from build123d import *

# Parameters (mm, degrees)
F0_W      = 25
F0_H      = 45
F1_DEPTH  = 25
F3_DEPTH  = 25
F5_DEPTH  = 25
F6_W      = 5
F6_H      = 12
F7_DEPTH  = 12
F9_DEPTH  = 25
F10_R     = 5
F11_W     = 5
F11_H     = 12
F12_DEPTH = 12
F14_DEPTH = 25
F15_R     = 5
F16_W     = 19
F16_H     = 6
F17_DEPTH = 19
F19_DEPTH = 12
F20_R     = 5
F21_R     = 5
F22_DEPTH = 2
F23_DEPTH = 19
F24_DEPTH = 7


with BuildPart() as f1:
    # F0 (on Front) → F1 (new body)
    with BuildSketch(Plane.XZ):
        with Locations((12.5, 22.5)):
            Rectangle(F0_W, F0_H)
    extrude(amount=F1_DEPTH)

    # F2 (on face) → F3 (cut)
    with BuildSketch(Plane.XZ.offset(25)):
        with BuildLine():
            ThreePointArc((16.5, 25), (9.6715728753, 27.8284271247), (12.5, 21))
            ThreePointArc((12.5, 21), (15.3284271247, 22.1715728753), (16.5, 25))
        make_face()
    extrude(amount=-F3_DEPTH, mode=Mode.SUBTRACT)

    # F4 (on face) → F5 (cut)
    with BuildSketch(Plane(origin=(0, 0, 0), x_dir=(0, -1, 0), z_dir=(-1, 0, 0))):
        with BuildLine():
            ThreePointArc((16.5, 37), (9.6715728753, 39.8284271247), (12.5, 33))
            ThreePointArc((12.5, 33), (15.3284271247, 34.1715728753), (16.5, 37))
        make_face()
    extrude(amount=-F5_DEPTH, mode=Mode.SUBTRACT)

    # F6 (on face) → F7 (join)
    with BuildSketch(Plane(origin=(0, 0, 0), x_dir=(0, -1, 0), z_dir=(-1, 0, 0))):
        with Locations((2.5, 31)):
            Rectangle(F6_W, F6_H)
    extrude(amount=F7_DEPTH)

    # F8 (on face) → F9 (cut)
    with BuildSketch(Plane.XZ.offset(5)):
        with BuildLine():
            ThreePointArc((-6, 33.5), (-8.5, 31), (-6, 28.5))
            Line((-6, 28.5), (-6, 33.5))
        make_face()
        with BuildLine():
            Line((-6, 33.5), (-6, 28.5))
            ThreePointArc((-6, 28.5), (-4.232233047, 29.232233047), (-3.5, 31))
            ThreePointArc((-3.5, 31), (-4.232233047, 32.767766953), (-6, 33.5))
        make_face()
    extrude(amount=-F9_DEPTH, mode=Mode.SUBTRACT)

    # F10
    f10_edges = [f1.edges().sort_by_distance(p)[0] for p in [
        (-12, -2.5, 37),
        (-12, -2.5, 25),
        (0, -2.5, 37),
    ]]
    fillet(f10_edges, radius=F10_R)

    # F11 (on face) → F12 (join)
    with BuildSketch(Plane.XZ.offset(25)):
        with Locations((22.5, 31)):
            Rectangle(F11_W, F11_H)
    extrude(amount=F12_DEPTH)

    # F13 (on face) → F14 (cut)
    with BuildSketch(Plane(origin=(20, 0, 0), x_dir=(0, -1, 0), z_dir=(-1, 0, 0))):
        with BuildLine():
            ThreePointArc((31, 33.5), (28.5, 31), (31, 28.5))
            Line((31, 28.5), (31, 33.5))
        make_face()
        with BuildLine():
            Line((31, 33.5), (31, 28.5))
            ThreePointArc((31, 28.5), (32.767766953, 29.232233047), (33.5, 31))
            ThreePointArc((33.5, 31), (32.767766953, 32.767766953), (31, 33.5))
        make_face()
    extrude(amount=-F14_DEPTH, mode=Mode.SUBTRACT)

    # F15
    f15_edges = [f1.edges().sort_by_distance(p)[0] for p in [
        (22.5, -37, 37),
        (22.5, -37, 25),
        (22.5, -25, 25),
    ]]
    fillet(f15_edges, radius=F15_R)

    # F16 (on face) → F17 (cut)
    with BuildSketch(Plane(origin=(0, 0, 0), x_dir=(0, -1, 0), z_dir=(-1, 0, 0))):
        with Locations((15.5, 7)):
            Rectangle(F16_W, F16_H)
    extrude(amount=-F17_DEPTH, mode=Mode.SUBTRACT)

    # F18 (on face) → F19 (cut)
    with BuildSketch(Plane(origin=(0, 0, 0), x_dir=(1, 0, 0), z_dir=(0, 0, -1))):
        Polygon((7.7781745931, 20.1085767529), (5.9480475741, 19.0519524259), (5.2781745931, 18.6652010799), (5.2781745931, 15.778449734), (7.7781745931, 14.335074061), (10.2781745931, 15.778449734), (10.2781745931, 18.6652010799), align=None)
    extrude(amount=-F19_DEPTH, mode=Mode.SUBTRACT)

    # F20
    f20_edges = [f1.edges().sort_by_distance(p)[0] for p in [
        (19, -6, 7),
    ]]
    fillet(f20_edges, radius=F20_R)

    # F21
    f21_edges = [f1.edges().sort_by_distance(p)[0] for p in [
        (0, -25, 2),
        (0, -25, 27.5),
    ]]
    fillet(f21_edges, radius=F21_R)

    # F22 (cut): a face of the model
    f22_faces = [f1.faces().sort_by_distance(p)[0] for p in [
        (12.59855993, -12.40144007, 45),
    ]]
    extrude(f22_faces, amount=-F22_DEPTH, mode=Mode.SUBTRACT)

    # F23 (cut): a face of the model
    f23_faces = [f1.faces().sort_by_distance(p)[0] for p in [
        (12.7730869211, -12.2269130789, 0),
    ]]
    extrude(f23_faces, amount=-F23_DEPTH, mode=Mode.SUBTRACT)

    # F24 (cut, through all): a face of the model
    f24_faces = [f1.faces().sort_by_distance(p)[0] for p in [
        (7.7781745931, -17.2218254069, 12),
    ]]
    extrude(f24_faces, amount=-F24_DEPTH, mode=Mode.SUBTRACT)


solid = f1.part
Could you check a few things on this model? Use its own coordinates, in mm. A direction names the side the tool comes from. Give positions to 0.01 mm unless a question says otherwise; leave off trailing zeros. Order: outer loops, then holes, each group sorted by start corner. A loop starts at its lowest first (then second) coordinate and runs counter-clockwise, first axis right, second up.
1. Which directions (+Z, -Z, +X, -X, +Y, -Y) give clear straight access to the entire face, cutting with the end or side of a thin tool? Please do faces 1 (the flat face through (22, -28, 37)), 2 (the flat face through (22, -31, 25)), 3 (the flat face through (-6, -2, 37)).
Answers below:
face 1: +Z, +X, -X, -Y
face 2: -Z, +X, -X, -Y
face 3: +Z, -X, +Y, -Y
2. I need wall thicknesses on L1, parallel to Z at x = 12.5, y = -12.75; L2, parallel to X at y = -18.75, z = 25; L3, parallel to Y at x = 7.75, z = 37. Which ranges of each line are inside material? Lowest first, please.
Answers below:
L1: z = 19 to 21, 29 to 33.01, 40.99 to 43
L2: x = 0 to 8.5, 16.5 to 25
L3: y = -25 to -16.5, -8.5 to 0
3. Suppose I cut it at B-B (x = -4.5). Write out the boundary of the cut face in (y, z).
Answers below:
outline: (-5, 25) - (0, 25) - (0, 29) - (-5, 29) - close; (-5, 33) - (0, 33) - (0, 37.03) - (-5, 37.03) - close
4. For pin 1 (4 mm diameter, centred on x = 23.5, y = -29.5, fed in from +Z); pin 2 (8 mm diameter, centred on x = 3.5, z = 33, fed in from -Y); pin 3 (6 mm diameter, centred on y = -15.5, z = 36, fed in from -X), each with a flat end and sliding along its axis, tell me the tip position at first contact or that it passes through.
Answers below:
pin 1: stops at z = 37
pin 2: stops at y = -25
pin 3: stops at x = 0
5. Suppose I cut it at A-A (y = -23). Write out the boundary of the cut face in (x, z).
Answers below:
outline: (1, 19) - (25, 19) - (25, 43) - (1, 43) - close; hole circle Ø8 at (12.5, 25)
6. Suppose I cut it at D-D (x = 5.5). Write out the boundary of the cut face in (y, z), plus the area to 3 significant figures.
Answers below:
outline: (-25, 19) - (0, 19) - (0, 43) - (-25, 43) - close; hole circle Ø8 at (-12.5, 37)
area: 550 mm2
7. Suppose I cut it at C-C (z = 30.5). Write out the boundary of the cut face in (x, y), plus the area to 3 significant figures.
Answers below:
outline: (-12, -5) - (-8.45, -5) - (-8.45, 0) - (-12, 0) - close; (-3.55, -5) - (0, -5) - (0, -20) arc R5 ccw to (5, -25) - (20, -25) - (20, -28.55) - (25, -28.55) - (25, 0) - (-3.55, 0) - close; (20, -37) - (25, -37) - (25, -33.45) - (20, -33.45) - close
area: 691 mm2
